```python
from build123d import *

# Parameters (mm, degrees)
SKETCH1_W           = 7
SKETCH1_H           = 7
BOSS_EXTRUDE1_DEPTH = 3
CUT_EXTRUDE1_DEPTH  = 7
CUT_EXTRUDE2_DEPTH  = 11
SKETCH4_R           = 1.8
CUT_EXTRUDE3_DEPTH  = 0.8
CUT_EXTRUDE4_DEPTH  = 0.4


with BuildPart() as part:
    # Sketch1 → Boss-Extrude1 (new body)
    with BuildSketch(Plane(origin=(0, 0, 0), x_dir=(1, 0, 0), z_dir=(0, 1, 0))):
        with Locations((3.5, 3.5)):
            Rectangle(SKETCH1_W, SKETCH1_H)
    extrude(amount=BOSS_EXTRUDE1_DEPTH)

    # Sketch2 → Cut-Extrude1 (cut)
    with BuildSketch(Plane.XY):
        Polygon((0, 0), (0.7, 3), (0, 3), align=None)
        Polygon((7, 0), (6.3, 3), (7, 3), align=None)
    extrude(amount=-CUT_EXTRUDE1_DEPTH, mode=Mode.SUBTRACT)

    # Sketch3 → Cut-Extrude2 (cut)
    with BuildSketch(Plane(origin=(0, 0, 0), x_dir=(0, 0, -1), z_dir=(1, 0, 0))):
        Polygon((0, 0), (0.7, 3), (0, 3), align=None)
        Polygon((7, 3), (6.3, 3), (7, 0), align=None)
    extrude(amount=CUT_EXTRUDE2_DEPTH, mode=Mode.SUBTRACT)

    # Sketch4 → Cut-Extrude3 (cut)
    with BuildSketch(Plane.XZ):
        with Locations(Location((3.5, -3.5, 0), (0, 0, 270))):
            Circle(SKETCH4_R)
    extrude(amount=-CUT_EXTRUDE3_DEPTH, mode=Mode.SUBTRACT)

    # Sketch5 → Cut-Extrude4 (cut)
    with BuildSketch(Plane(origin=(0, 3, 0), x_dir=(1, 0, 0), z_dir=(0, 1, 0))):
        with BuildLine():
            Line((4.301123745, 3.0403235), (4.974200669, 2.815964526))
            add(Edge.make_bspline(
                [(4.974200669, 2.815964526), (4.960521674, 2.771832567), (4.933733899, 2.68540831), (4.884547054, 2.561541828), (4.828302659, 2.446749112), (4.767023387, 2.33968659), (4.696898403, 2.243120033), (4.621853673, 2.15385218), (4.53965782, 2.073763183), (4.45071642, 2.002682023), (4.355885584, 1.939823406), (4.25406375, 1.886683329), (4.146770466, 1.840915158), (4.032917717, 1.803833291), (3.913261107, 1.774136343), (3.787239198, 1.754521348), (3.655441508, 1.741221733), (3.565448152, 1.739779731), (3.519372944, 1.739041449)],
                knots=[0, 0, 0, 0, 1.126640671, 2.206316847, 3.246446654, 4.24268115, 5.210795778, 6.153057602, 7.084219323, 8.004711971, 8.926421631, 9.854560063, 10.802134612, 11.768317461, 12.772025444, 13.805668576, 14.876536225, 16, 16, 16, 16], degree=3))
            add(Edge.make_bspline(
                [(3.519372944, 1.739041449), (3.462502515, 1.740217406), (3.350636682, 1.742530549), (3.187043495, 1.765815525), (3.031146586, 1.80214564), (2.882722932, 1.852444053), (2.742763243, 1.919064174), (2.609990608, 1.999266162), (2.485371298, 2.094678249), (2.3693425, 2.203692372), (2.263927531, 2.325476328), (2.172770854, 2.459372031), (2.094880625, 2.603493215), (2.031925726, 2.758527068), (1.982699244, 2.924314395), (1.948215991, 3.100625971), (1.926638564, 3.287517332), (1.924180264, 3.415596421), (1.922918617, 3.481329109)],
                knots=[0, 0, 0, 0, 1.025049111, 2.016302254, 2.973197159, 3.90886983, 4.83646737, 5.763135642, 6.70136783, 7.661478232, 8.629732022, 9.600038443, 10.576877021, 11.5787097, 12.612181225, 13.690866959, 14.814907849, 16, 16, 16, 16], degree=3))
            add(Edge.make_bspline(
                [(1.922918617, 3.481329109), (1.924174578, 3.550566485), (1.926624727, 3.685635974), (1.948242577, 3.882015446), (1.981803001, 4.067091651), (2.031112683, 4.239717041), (2.09314245, 4.401106495), (2.171127245, 4.549657913), (2.261374638, 4.687351889), (2.366311182, 4.811664664), (2.482868768, 4.922037599), (2.607774637, 5.019637111), (2.74219405, 5.101516105), (2.885391432, 5.168472462), (3.037558838, 5.220286586), (3.198396842, 5.257596822), (3.368037039, 5.279313779), (3.484020884, 5.282359114), (3.543211085, 5.283913244)],
                knots=[0, 0, 0, 0, 1.212648312, 2.365655595, 3.457000981, 4.504219827, 5.506356588, 6.480637568, 7.437950897, 8.385265166, 9.323599949, 10.245787653, 11.157260172, 12.074946661, 13.00980897, 13.968233668, 14.963125779, 16, 16, 16, 16], degree=3))
            add(Edge.make_bspline(
                [(3.543211085, 5.283913244), (3.594904175, 5.282610712), (3.696255358, 5.280056925), (3.844673873, 5.262706402), (3.98533309, 5.232257393), (4.118993318, 5.191158002), (4.244893689, 5.136917739), (4.363259754, 5.070636697), (4.474498364, 4.992665569), (4.541521917, 4.931760883), (4.575262367, 4.901100744)],
                knots=[0, 0, 0, 0, 1.098510076, 2.153775193, 3.169777012, 4.153122333, 5.120892526, 6.076995459, 7.031936742, 8, 8, 8, 8], degree=3))
            add(Edge.make_bspline(
                [(4.575262367, 4.901100744), (4.594817889, 4.881591385), (4.634388278, 4.842114408), (4.687225854, 4.775466084), (4.73732244, 4.703719152), (4.783882904, 4.625649701), (4.825435673, 4.54066776), (4.863980304, 4.45007838), (4.8994669, 4.353532371), (4.919201528, 4.286342314), (4.929328874, 4.251861961)],
                knots=[0, 0, 0, 0, 0.885292881, 1.791380647, 2.722937556, 3.69093542, 4.703306561, 5.754477758, 6.847650944, 8, 8, 8, 8], degree=3))
            Line((4.929328874, 4.251861961), (4.256251951, 4.117246577))
            add(Edge.make_bspline(
                [(4.256251951, 4.117246577), (4.250531073, 4.139323539), (4.239262446, 4.182809362), (4.216461913, 4.245296102), (4.190307903, 4.304590437), (4.157892404, 4.359240043), (4.123458761, 4.411676126), (4.082691271, 4.459570361), (4.038193489, 4.504177952), (3.98964486, 4.545035979), (3.937624153, 4.581318844), (3.883132951, 4.61393488), (3.825180855, 4.640559757), (3.76453877, 4.66209922), (3.701448228, 4.680158437), (3.63534753, 4.691314457), (3.566804403, 4.699878675), (3.520103543, 4.700342739), (3.496235925, 4.70057991)],
                knots=[0, 0, 0, 0, 1.051226935, 2.070641259, 3.064374968, 4.034983734, 4.997599858, 5.953980297, 6.92954377, 7.901109626, 8.875958313, 9.851998019, 10.826131395, 11.811470594, 12.818270757, 13.847890818, 14.900111925, 16, 16, 16, 16], degree=3))
            add(Edge.make_bspline(
                [(3.496235925, 4.70057991), (3.463458178, 4.699917949), (3.399485824, 4.698625999), (3.305980427, 4.684221631), (3.216859157, 4.664118846), (3.132481433, 4.633421996), (3.053369786, 4.594160979), (2.978625107, 4.546434822), (2.908657635, 4.490447949), (2.843443721, 4.425537099), (2.784923098, 4.350528652), (2.733475117, 4.265267743), (2.690794404, 4.168786384), (2.656144454, 4.062031362), (2.628870995, 3.944748811), (2.609395598, 3.81678831), (2.598625118, 3.678062323), (2.596890981, 3.582075039), (2.59599554, 3.532511)],
                knots=[0, 0, 0, 0, 0.938194206, 1.831074359, 2.704771284, 3.551924377, 4.396294915, 5.230222094, 6.087631332, 6.958733431, 7.860107878, 8.806247581, 9.804197948, 10.875520245, 12.017191412, 13.250061517, 14.580040491, 16, 16, 16, 16], degree=3))
            add(Edge.make_bspline(
                [(2.59599554, 3.532511), (2.596882163, 3.479909852), (2.598590549, 3.378555543), (2.609358744, 3.232361327), (2.628958677, 3.097901323), (2.655869672, 2.974936912), (2.690694237, 2.863543412), (2.733302771, 2.763913587), (2.783956188, 2.675930758), (2.84257568, 2.599653514), (2.907679246, 2.534131595), (2.977503606, 2.477797664), (3.05163681, 2.429632374), (3.130524959, 2.39000508), (3.2144681, 2.360027472), (3.302776345, 2.338287186), (3.395773712, 2.32446654), (3.459494346, 2.323081807), (3.492029194, 2.322374782)],
                knots=[0, 0, 0, 0, 1.475208372, 2.842499301, 4.107722225, 5.282836115, 6.369007568, 7.375918121, 8.315702116, 9.208439171, 10.065831443, 10.90006451, 11.71996243, 12.54067204, 13.369972975, 14.214060185, 15.088124569, 16, 16, 16, 16], degree=3))
            add(Edge.make_bspline(
                [(3.492029194, 2.322374782), (3.516116809, 2.32297573), (3.563481527, 2.324157405), (3.633490233, 2.331657405), (3.700684312, 2.345970073), (3.765392659, 2.364895987), (3.827866687, 2.388642426), (3.887153461, 2.419104331), (3.944419425, 2.454115768), (3.998476353, 2.495146489), (4.050048096, 2.541211307), (4.097084586, 2.594450756), (4.140714836, 2.653585613), (4.180385329, 2.719011076), (4.217421584, 2.790167129), (4.248932218, 2.868162419), (4.278287198, 2.951736508), (4.293378607, 3.010278741), (4.301123745, 3.0403235)],
                knots=[0, 0, 0, 0, 0.980177776, 1.927374078, 2.859849964, 3.771585772, 4.668674471, 5.574490016, 6.479656464, 7.396337719, 8.332153134, 9.288470092, 10.28125149, 11.318486971, 12.398724812, 13.541284404, 14.738150009, 16, 16, 16, 16], degree=3))
        make_face()
    extrude(amount=-CUT_EXTRUDE4_DEPTH, mode=Mode.SUBTRACT)


solid = part.part
```
Source: CAD feature listing. Evaluate the final solid. Frame: model axes, mm. A direction names the side the tool comes from. Coordinates: 2 decimals unless noted, no trailing zeros. Write each loop counter-clockwise with the first axis right and the second up, starting at its lowest first coordinate (ties: lowest second). Pieces come first, ordered by that corner, then holes. Notation, with made-up numbers: (64, -35) - (123, -35) arc R9 cw to (123, -27) - close; hole circle Ø10 at (13, 72.5). An arc over 180 degrees is marked (long way). Answer as a JSON object with one key per item and string values.
Q1. Material intervals for line 1 (Y direction, x = 5, z = -4); line 2 (X direction, y = 0.3, z = -3.5); line 3 (Z direction, x = 1, y = 0.65), sorted ascending. Write a range as [from, to].
Ans:
{"line 1": "y = [0.8, 3]", "line 2": "x = [0.07, 1.7], [5.3, 6.93]", "line 3": "z = [-6.85, -0.15]"}
Q2. Section query A-A, the plane y = 0.7. Output: boundary loops of the cut face in (x, z), plus the area to 3 significant figures.
Ans:
{"outline": "(0.16, -6.84) - (6.84, -6.84) - (6.84, -0.16) - (0.16, -0.16) - close; hole circle Ø3.6 at (3.5, -3.5)", "area": "34.4 mm2"}
Q3. Section query B-B, the plane y = 1.8. Output: boundary loops of the cut face in (x, z).
Ans:
{"outline": "(0.42, -6.58) - (6.58, -6.58) - (6.58, -0.42) - (0.42, -0.42) - close"}
Q4. Set-up query: faces 1 (the flat face through (3.451, 1.479, -0.345)), 2 (the flat face through (2.45, 2.6, -3.93)). Return all of +Z, -Z, +X, -X, +Y, -Y with unobstructed straight access to the full face (end or side cutting, diameter ignored); none if empty.
Ans:
{"face 1": "+Z, +X, -X, +Y", "face 2": "+Y"}
Q5. Section query D-D, the plane y = 0.2. Output: boundary loops of the cut face in (x, z).
Ans:
{"outline": "(0.05, -6.95) - (6.95, -6.95) - (6.95, -0.05) - (0.05, -0.05) - close; hole circle Ø3.6 at (3.5, -3.5)"}
Q6. First-contact query: pin 1 Ø1.5 at (y, z) = (0.5, -5) entering from -X; pin 2 Ø1.8 at (x, z) = (3.5, -3.5) entering from -Y; pin 3 Ø1.5 at (y, z) = (2.5, -4) entering from +X. Flat tips, straight axial feed; report the tip coordinate or a pass-through.
Ans:
{"pin 1": "stops at x = 0", "pin 2": "stops at y = 0.8", "pin 3": "stops at x = 6.59"}
Q7. Draft query along X for faces 3 (the cylindrical face through (4.041, 0.394, -5.217)), 4 (the flat face through (0.345, 1.479, -3.451)), 5 (the flat face through (2, 0, -5)), 6 (the flat face through (4, 0.8, -3)). Return one class per face: released by +X, released by -X, zero draft, split by the parting line, or undercut.
Ans:
{"face 3": "undercut", "face 4": "released by -X", "face 5": "zero draft", "face 6": "undercut"}
Q8. Section query C-C, the plane x = 5.75. Output: boundary loops of the cut face in (y, z), plus the area to 3 significant figures.
Ans:
{"outline": "(0, -7) - (3, -6.3) - (3, -0.7) - (0, 0) - close", "area": "18.9 mm2"}
